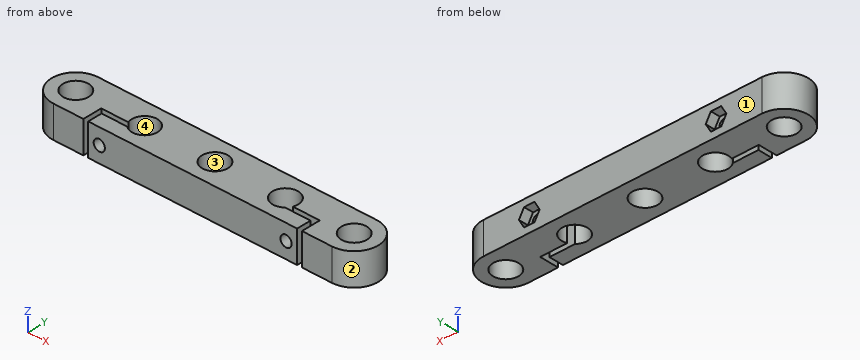
Autodesk Inventor part; units mm, degrees
ref_plane "YZ Plane" through (0, 0, 0) normal (1, 0, 0) x (0, 1, 0)
ref_plane "XZ Plane" through (0, 0, 0) normal (0, 1, 0) x (-1, 0, 0)
ref_plane "XY Plane" through (0, 0, 0) normal (0, 0, 1) x (1, 0, 0)
sketch "Sketch1" plane through (0, 0, 0) normal (0, 0, 1) x (1, 0, 0)
  circle A0 centre (0, 0) radius 4
  circle A1 centre (43.5, 0) radius 4
  circle A2 centre (22, 0) radius 4
  line L0 (0, 0) -> (43.5, 0) construction
  line L1 (0, -7.5) -> (43.5, -7.5)
  line L2 (43.5, 7.5) -> (0, 7.5)
  arc A3 (0, 7.5) -> (0, -7.5) centre (0, 0) ccw
  arc A4 (43.5, -7.5) -> (43.5, 7.5) centre (43.5, 0) ccw
  point P0 (21.75, 0)
  dimension "d1" = 8
  dimension "d2" = 8
  dimension "d4" = 15
  dimension "d19" = 43.5
  dimension "d22" = 22
extrude "Extrusion1" add sketch "Sketch1" along normal blind 10
sketch "Sketch2" plane through (0, 0, 10) normal (0, 0, 1) x (1, 0, 0)
  line L0 (24.6458, -1.5) -> (34.1458, -1.5)
  line L1 (34.1458, -1.5) -> (34.1458, -3)
  line L2 (34.1458, -3) -> (24.6458, -3)
  line L3 (24.6458, -3) -> (24.6458, -1.5)
  line L4 (0, -7.5) -> (43.5, -7.5)
  line L5 (34.1458, -3) -> (32.6458, -3)
  line L6 (32.6458, -3) -> (32.6458, -7.5)
  line L7 (32.6458, -7.5) -> (34.1458, -7.5)
  line L8 (34.1458, -7.5) -> (34.1458, -3)
  circle A0 centre (22, 0) radius 4 construction
  point P0 (0, 0)
  dimension "d7" = 1.5
  dimension "d8" = 8
  dimension "d9" = 1.5
  dimension "d18" = 1
extrude "Extrusion2" cut sketch "Sketch2" against normal through all
sketch "Sketch3" plane through (0, -7.5, 0) normal (0, -1, 0) x (1, 0, 0)
  line L0 (24.6458, 0) -> (32.6458, 0) construction
  line L1 (24.6458, 10) -> (24.6458, 0) construction
  line L2 (32.6458, 10) -> (24.6458, 10) construction
  line L3 (32.6458, 10) -> (32.6458, 0) construction
  line L4 (32.6458, 5) -> (25.7081, 5) construction
  line L5 (25.7081, 0) -> (25.7081, 10) construction
  circle A0 centre (29.1769, 5) radius 1.75
  point P0 (0, 0)
  dimension "d12" = 3.5
extrude "Extrusion3" cut sketch "Sketch3" against normal through all
sketch "Sketch4" plane through (0, 7.5, 0) normal (0, 1, 0) x (1, 0, 0)
  circle A0 centre (29.1769, -5) radius 1.75 construction
  line L0 (30.7935, -2.2) -> (32.4101, -5)
  line L1 (32.4101, -5) -> (30.7935, -7.8)
  line L2 (30.7935, -7.8) -> (27.5603, -7.8)
  line L3 (27.5603, -7.8) -> (25.9438, -5)
  line L4 (25.9438, -5) -> (27.5603, -2.2)
  line L5 (27.5603, -2.2) -> (30.7935, -2.2)
  point P0 (0, 0)
  dimension "d15" = 5.6
extrude "Extrusion4" cut sketch "Sketch4" against normal blind 3
mirror "Mirror1" about plane through (0, 0, 0) normal (1, 0, 0) of "Extrusion1", "Extrusion2", "Extrusion3", "Extrusion4"
properties part number "guide rod mount"
Here's how the part is built. I have some questions about the finished solid (model axes, mm). Face numbers are marked on the shaded views. Give positions to 0.01 mm unless a question says otherwise; leave off trailing zeros. Order: outer loops, then holes, each group sorted by start corner. A loop starts at its lowest first (then second) coordinate and runs counter-clockwise, first axis right, second up. Notation, with made-up numbers: (43.25, 76.25) - (100.25, 76.25) arc R24 cw to (100.25, 114.25) - close; hole circle Ø8 at (25.25, -24.5). An arc over 180 degrees is marked (long way). Answer as a JSON object with one key per item and string values. Group by question number.
Item 1: If we section it at D-D on x = 23: Please give me the cut outline in (y, z).
Item 2: If we section it at B-B on x = -22: Please give me the cut outline in (y, z).
Item 3: If we section it at C-C on y = -5.75: Please give me the cut outline in (x, z).
Item 4: If we section it at A-A on y = 0: Please give me the cut outline in (x, z).
Item 5: Please list where these lines run through material, in increasing order: probe 1 along X at (y, z) = (6.5, 7); probe 2 along X at (y, z) = (-5.25, 4); probe 3 along Y at (x, z) = (-30.5, 1).
Item 6: For P1, Ø6.5, axis at x = 0, y = 0, coming from the -Z side; P2, Ø5, axis at y = -6, z = 5.5, coming from the +X side; P3, Ø5.5, axis at x = -29.18, z = 5, coming from the +Y side, each with a flat end and sliding along its axis, tell me the tip position at first contact or that it passes through.
Item 7: If we mould it in two halves opening along X, with no side actions, what happens to the marked faces 1, 2, 3 and 4? For each: pulls with the +X half, pulls with the -X half, needs draft (parallel to the pull), parting line crosses it, or undercut.
Result set:
{
 "1": {"outline": "(-7.5, 0) - (-3.87, 0) - (-3.87, 10) - (-7.5, 10) - close; (3.87, 0) - (7.5, 0) - (7.5, 10) - (3.87, 10) - close"},
 "2": {"outline": "(-7.5, 0) - (-4, 0) - (-4, 10) - (-7.5, 10) - close; (4, 0) - (7.5, 0) - (7.5, 10) - (4, 10) - close"},
 "3": {"outline": "(-48.32, 0) - (-34.15, 0) - (-34.15, 10) - (-48.32, 10) - close; (-32.65, 0) - (32.65, 0) - (32.65, 10) - (-32.65, 10) - close; (34.15, 0) - (48.32, 0) - (48.32, 10) - (34.15, 10) - close; hole circle Ø3.5 at (-29.18, 5); hole circle Ø3.5 at (29.18, 5)"},
 "4": {"outline": "(-51, 0) - (-47.5, 0) - (-47.5, 10) - (-51, 10) - close; (-39.5, 0) - (-26, 0) - (-26, 10) - (-39.5, 10) - close; (-18, 0) - (-4, 0) - (-4, 10) - (-18, 10) - close; (4, 0) - (18, 0) - (18, 10) - (4, 10) - close; (26, 0) - (39.5, 0) - (39.5, 10) - (26, 10) - close; (47.5, 0) - (51, 0) - (51, 10) - (47.5, 10) - close; hole circle Ø3.5 at (-29.18, 5); hole circle Ø3.5 at (29.18, 5)"},
 "5": {"probe 1": "-47.24 to -31.26, -27.1 to 27.1, 31.26 to 47.24", "probe 2": "-48.86 to -34.15, -32.65 to -30.61, -27.74 to 27.74, 30.61 to 32.65, 34.15 to 48.86", "probe 3": "-7.5 to -3, -1.5 to 7.5"},
 "6": {"P1": "through", "P2": "x = 50.13", "P3": "y = 4.5"},
 "7": {"face 1": "needs draft", "face 2": "pulls with the +X half", "face 3": "undercut", "face 4": "undercut"}
}
